from build123d import *

# Parameters (mm, degrees)
SKETCH_1_R      = 5
EXTRUDE_1_DEPTH = 15
FILLET_1_R      = 1


with BuildPart() as part:
    # 草图1 → 凸台-拉伸1 (new body)
    with BuildSketch(Plane.XY):
        with BuildLine():
            Line((15, 2.5), (25, 2.5))
            Line((25, 2.5), (25, -2.5))
            Line((25, -2.5), (-25, -2.5))
            Line((-25, -2.5), (-25, 2.5))
            Line((-25, 2.5), (-15, 2.5))
            Line((-15, 2.5), (-15, 12.5))
            ThreePointArc((-15, 12.5), (0, 27.5), (15, 12.5))
            Line((15, 12.5), (15, 2.5))
        make_face()
        with Locations((0, 12.5)):
            Circle(SKETCH_1_R, mode=Mode.SUBTRACT)
    extrude(amount=EXTRUDE_1_DEPTH)

    # 圆角1
    fillet_1_edges = [part.edges().sort_by_distance(p)[0] for p in [
        (-25, 2.5, 7.5),
        (25, 2.5, 7.5),
    ]]
    fillet(fillet_1_edges, radius=FILLET_1_R)


solid = part.part
Could you check a few things on this model? Use its own coordinates, in mm. A direction names the side the tool comes from. Coordinates: 2 decimals unless noted, no trailing zeros. Order: outer loops, then holes, each group sorted by start corner. A loop starts at its lowest first (then second) coordinate and runs counter-clockwise, first axis right, second up.
Q1. Which directions (+Z, -Z, +X, -X, +Y, -Y) give clear straight access to the entire face, cutting with the end or side of a thin tool? Please do faces 4 (the flat face through (25, 0, 7)), 5 (the flat face through (19, 2.5, 7)), 6 (the flat face through (-15, 7, 7)).
Q2. Will these pins go through, and if not, where does the flat tip stop? pin 1 (8 mm diameter, centred on x = 15.5, z = 11.5, fed in from +Y); pin 2 (3 mm diameter, centred on y = 6.5, z = 9, fed in from -X); pin 3 (3 mm diameter, centred on y = 17, z = 8.5, fed in from -X); pin 4 (2 mm diameter, centred on y = 2, z = 8, fed in from -X).
Q3. Please list where these lines run through material, in increasing order: L1, parallel to Y at x = 0, z = 8; L2, parallel to X at y = 7.25, z = 4; L3, parallel to Y at x = -18.5, z = 5.75.
Q4. Suppose I cut it at D-D on x = 17. Please give me the cut outline in (y, z).
Q5. Suppose I cut it at C-C on y = 21.5. Please give me the cut outline in (x, z), and give its area (3 significant figures).
Q6. Thinking about a two-plate mould opening in Y: for faces 1 (the cylindrical face through (-24.715, 2.199, 7.605)), 2 (the flat face through (-25, -1, 7)), 3 (the cylindrical face through (-0.651, 17.457, 7.395)), which applies, released by +Y, released by -Y, zero draft, split by the parting line, or undercut?
Q7. Suppose I cut it at A-A on x = 0. Please give me the cut outline in (y, z), and give its area (3 significant figures).
Q8. Suppose I cut it at B-B on y = 11.25. Please give me the cut outline in (x, z).
Answer:
1. face 4: +Z, -Z, +X, +Y, -Y
1. face 5: +Z, -Z, +X, +Y
1. face 6: +Z, -Z, -X, +Y
2. pin 1: stops at y = 22.13
2. pin 2: stops at x = -15
2. pin 3: stops at x = -14.7
2. pin 4: stops at x = -25
3. L1: y = -2.5 to 7.5, 17.5 to 27.5
3. L2: x = -15 to 15
3. L3: y = -2.5 to 2.5
4. outline: (-2.5, 0) - (2.5, 0) - (2.5, 15) - (-2.5, 15) - close
5. outline: (-12, 0) - (12, 0) - (12, 15) - (-12, 15) - close
5. area: 360 mm2
6. face 1: released by +Y
6. face 2: zero draft
6. face 3: undercut
7. outline: (-2.5, 0) - (7.5, 0) - (7.5, 15) - (-2.5, 15) - close; (17.5, 0) - (27.5, 0) - (27.5, 15) - (17.5, 15) - close
7. area: 300 mm2
8. outline: (-15, 0) - (-4.84, 0) - (-4.84, 15) - (-15, 15) - close; (4.84, 0) - (15, 0) - (15, 15) - (4.84, 15) - close
